from build123d import *

# Parameters (mm, degrees)
BOSS_EXTRUDE3_START = 4.7625
SKETCH2_R           = 3.175
BOSS_EXTRUDE3_DEPTH = 2.54


with BuildPart() as part:
    # Sketch2 → Boss-Extrude3 (new body)
    with BuildSketch(Plane.XY.offset(BOSS_EXTRUDE3_START)):
        with BuildLine():
            Line((111.752654756, -67.172007853), (131.648348491, -84.372647625))
            ThreePointArc((131.648348491, -84.372647625), (113.938329585, -85.444576189), (114.582474398, -103.175308774))
            Line((114.582474398, -103.175308774), (95.540074367, -85.034535944))
            ThreePointArc((95.540074367, -85.034535944), (94.928136795, -68.190339989), (111.752654756, -67.172007853))
        make_face()
        with Locations((103.862003689, -76.298992609)):
            Circle(SKETCH2_R, mode=Mode.SUBTRACT)
    extrude(amount=BOSS_EXTRUDE3_DEPTH)


solid = part.part
Geometry: final body of the model. Coordinates: model frame, mm. Give positions to 0.01 mm unless a question says otherwise; leave off trailing zeros. Write each loop counter-clockwise with the first axis right and the second up, starting at its lowest first coordinate (ties: lowest second). Pieces come first, ordered by that corner, then holes. Notation, with made-up numbers: (55.5, -9.5) - (91.5, -9.5) arc R8 cw to (91.5, -1.5) - close; hole circle Ø1 at (-37, 49). An arc over 180 degrees is marked (long way). Return JSON: item names as keys, results as strings. Group by question number.
1) Line query: line 1 (X direction, y = -74.5, z = 6.5); line 2 (X direction, y = -79, z = 6.3); line 3 (Y direction, x = 101, z = 6.95). Output: solid intervals per line, ascending.
2) Mould query, pull axis X, two halves, no side actions, for faces 1 (the flat face through (121.56, -75.65, 6.01)), 2 (the flat face through (108, -79, 4.762)), 3 (the cylindrical face through (114.13, -85.24, 6.01)), 4 (the cylindrical face through (94.75, -68.39, 6.01)). Classes: released by +X, released by -X, zero draft, split by the parting line, or undercut.
3) Section B-B on z = 6.35. Return the cut outline in (x, y) (3 decimals), plus the area to 3 significant figures.
4) First-contact query: P1, Ø1, axis at y = -68, z = 6.5, coming from the -X side. Flat tip, straight axial feed; report the tip coordinate or a pass-through.
5) Section A-A on y = -78. Return the cut outline in (x, z).
6) Section C-C on x = 120. Return the cut outline in (y, z).
7) Section D-D on y = -97. Return the cut outline in (x, z).
Filled in:
{
 "1": {"line 1": "x = 91.93 to 101.25, 106.48 to 120.23", "line 2": "x = 92.1 to 102.19, 105.53 to 125.43", "line 3": "y = -90.24 to -77.67, -74.92 to -64.58"},
 "2": {"face 1": "released by +X", "face 2": "zero draft", "face 3": "undercut", "face 4": "split by the parting line"},
 "3": {"outline": "(95.54, -85.035) - (114.582, -103.175) arc R12.7 cw to (131.648, -84.373) - (111.753, -67.172) arc R12.065 ccw to start; hole circle Ø6.35 at (103.862, -76.299)", "area": "595 mm^2"},
 "4": {"P1": "stops at x = 94.66"},
 "5": {"outline": "(91.92, 4.76) - (101.18, 4.76) - (101.18, 7.3) - (91.92, 7.3) - close; (106.54, 4.76) - (124.28, 4.76) - (124.28, 7.3) - (106.54, 7.3) - close"},
 "6": {"outline": "(-81.73, 4.76) - (-74.3, 4.76) - (-74.3, 7.3) - (-81.73, 7.3) - close"},
 "7": {"outline": "(108.1, 4.76) - (111.01, 4.76) - (111.01, 7.3) - (108.1, 7.3) - close"}
}
